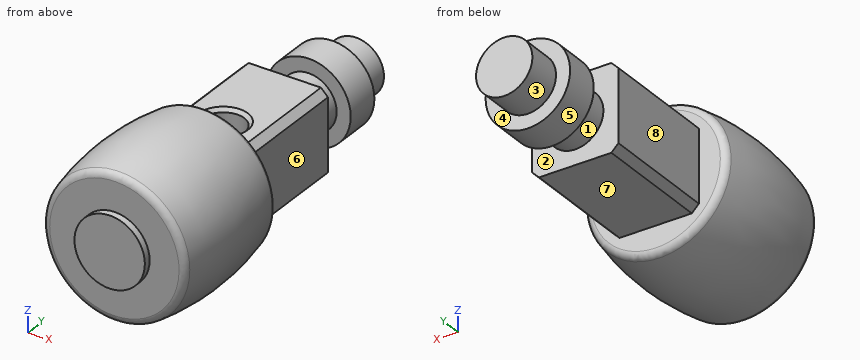
```python
from build123d import *

# Parameters (mm, degrees)
SKETCH2_OUTSIDE_W   = 35.948
SKETCH2_OUTSIDE_H   = 35.948
CUT_EXTRUDE1_DEPTH  = 17
SKETCH3_R           = 3
CUT_EXTRUDE2_DEPTH  = 8.269428
CHAMFER1_SIZE       = 0.5
SKETCH4_R           = 5
BOSS_EXTRUDE1_DEPTH = 1
FILLET1_R           = 1


with BuildPart() as part:
    # Sketch1 → Revolve1 (revolve)
    with BuildSketch(Plane.XY):
        with BuildLine():
            Line((0, 0), (0, 51))
            Line((0, 51), (4, 51))
            Line((4, 51), (4, 46.000706479))
            Line((4, 46.000706479), (6, 46.000706479))
            Line((6, 46.000706479), (6, 40.999293521))
            Line((6, 40.999293521), (4, 40.999293521))
            Line((4, 40.999293521), (4, 36))
            Line((4, 36), (8, 36))
            Line((8, 36), (8, 19))
            Line((8, 19), (10, 19))
            ThreePointArc((10, 19), (11, 9.5), (10, 0))
            Line((10, 0), (0, 0))
        make_face()
    revolve(axis=Axis((0, 0, 0), (0, 1, 0)))

    # Sketch2 outside → Cut-Extrude1 (cut)
    with BuildSketch(Plane(origin=(0, 36, 0), x_dir=(1, 0, 0), z_dir=(0, 1, 0))):
        Rectangle(SKETCH2_OUTSIDE_W, SKETCH2_OUTSIDE_H)
        Polygon((-6.134713835, 5.134713835), (-5.134713835, 6.134713835), (5.134713835, 6.134713835), (6.134713835, 5.134713835), (6.134713835, -5.134713835), (5.134713835, -6.134713835), (-5.134713835, -6.134713835), (-6.134713835, -5.134713835), align=None, mode=Mode.SUBTRACT)
    extrude(amount=-CUT_EXTRUDE1_DEPTH, mode=Mode.SUBTRACT)

    # Sketch3 → Cut-Extrude2 (cut)
    with BuildSketch(Plane.XY.offset(6.134713835)):
        with Locations((0.000286165, 23)):
            Circle(SKETCH3_R)
    extrude(amount=-CUT_EXTRUDE2_DEPTH, mode=Mode.SUBTRACT)

    # Chamfer1
    chamfer1_edges = [part.edges().sort_by_distance(p)[0] for p in [
        (-2.999713835, 23, 6.134713835),
    ]]
    chamfer(chamfer1_edges, length=CHAMFER1_SIZE)

    # Sketch4 → Boss-Extrude1 (add)
    with BuildSketch(Plane.XZ):
        Circle(SKETCH4_R)
    extrude(amount=BOSS_EXTRUDE1_DEPTH)

    # Fillet1
    fillet1_edges = [part.edges().sort_by_distance(p)[0] for p in [
        (-10, 0, 0),
        (-10, 19, 0),
    ]]
    fillet(fillet1_edges, radius=FILLET1_R)


solid = part.part
```
Design review of the part built by this model. Coordinates are the model's own, in mm. Face numbers are marked on the shaded views. A direction names the side the tool comes from. Give positions to 0.01 mm unless a question says otherwise; leave off trailing zeros. Write each loop counter-clockwise with the first axis right and the second up, starting at its lowest first coordinate (ties: lowest second). Pieces come first, ordered by that corner, then holes.
(1) Mouldability with a two-part tool opening along Y and no side actions: class the marked faces 1, 2, 3 and 4 as +Y half, -Y half, draft (parallel to the pull), parting line (faces both ways), or undercut.
Checked values:
face 1: undercut
face 2: undercut
face 3: draft
face 4: +Y half
(2) Clearance check with flat-ended pins moving along their axes: pin 1 Ø5 at (x, y) = (-1, 26.5) entering from +Z; pin 2 Ø3 at (y, z) = (6, 4.5) entering from +X; pin 3 Ø12 at (x, y) = (1, 23.5) entering from +Z. State where each tip first meets the part, or that it passes through.
Checked values:
pin 1: stops at z = 6.13
pin 2: stops at x = 10.46
pin 3: stops at z = 10.28
(3) Tool access review of the marked faces 5, 6, 7 and 8: name each direction out of +Z, -Z, +X, -X, +Y, -Y from which nothing blocks a thin tool from reaching the whole face with its end or side.
Checked values:
face 5: +Y
face 6: +Z, -Z, +X, +Y
face 7: -Z, +X, -X, +Y
face 8: +Z, -Z, -X, +Y
(4) Add section A-A (y = 34). Give the boundary of the cut face in (x, z), and give its area (3 significant figures).
Checked values:
outline: (-6.13, -5.13) - (-5.13, -6.13) - (5.13, -6.13) - (6.13, -5.13) - (6.13, 5.13) - (5.13, 6.13) - (-5.13, 6.13) - (-6.13, 5.13) - close
area: 149 mm2
(5) Wall thickness on line 1 along Y through (x, z) = (-1.5, 5.5); line 2 along Y through (x, z) = (2.5, -4.5); line 3 along Y through (x, z) = (-1.25, 4): over which ranges is each line inside the solid? List them lowest first.
Checked values:
line 1: y = 0 to 20.4, 25.6 to 36, 41 to 46
line 2: y = 0 to 36, 41 to 46
line 3: y = -1 to 20.27, 25.73 to 36, 41 to 46
(6) Add section B-B (y = 23). Give the boundary of the cut face in (x, z).
Checked values:
outline: (-6.13, -5.13) - (-5.13, -6.13) - (5.13, -6.13) - (6.13, -5.13) - (6.13, 5.13) - (5.13, 6.13) - (3.5, 6.13) - (3, 5.63) - (3, -2.13) - (-3, -2.13) - (-3, 5.63) - (-3.5, 6.13) - (-5.13, 6.13) - (-6.13, 5.13) - close
